```python
from build123d import *

# Parameters (mm, degrees)
BOSS_EXTRUDE1_DEPTH = 160
FILLET1_R           = 10


with BuildPart() as part:
    # Sketch1 → Boss-Extrude1 (new body)
    with BuildSketch(Plane.XY):
        with BuildLine():
            Line((0, 0), (0, -254))
            ThreePointArc((0, -254), (-1.757359313, -258.242640687), (-6, -260))
            Line((-6, -260), (-80, -260))
            Line((-80, -260), (-80, -254))
            Line((-80, -254), (-8, -254))
            ThreePointArc((-8, -254), (-6.585786438, -253.414213562), (-6, -252))
            Line((-6, -252), (-6, 0))
            Line((-6, 0), (0, 0))
        make_face()
    extrude(amount=BOSS_EXTRUDE1_DEPTH)

    # Fillet1
    fillet1_edges = [part.edges().sort_by_distance(p)[0] for p in [
        (-3, 0, 0),
        (-80, -257, 160),
        (-3, 0, 160),
        (-80, -257, 0),
    ]]
    fillet(fillet1_edges, radius=FILLET1_R)


solid = part.part
```
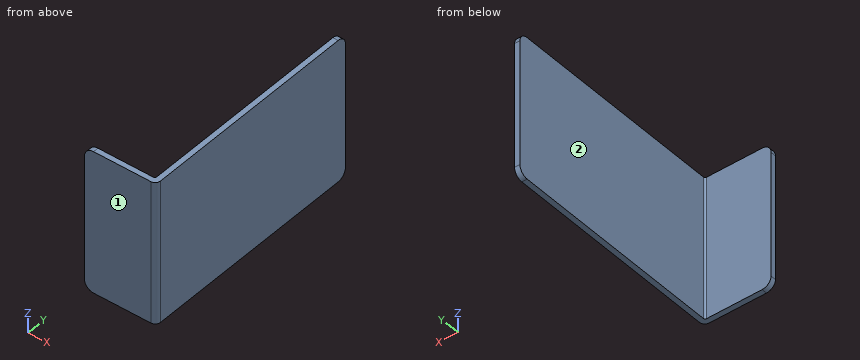
Could you check a few things on this model? Use its own coordinates, in mm. Face numbers are marked on the shaded views. A direction names the side the tool comes from. Coordinates: 2 decimals unless noted, no trailing zeros. Order: outer loops, then holes, each group sorted by start corner. A loop starts at its lowest first (then second) coordinate and runs counter-clockwise, first axis right, second up. Notation, with made-up numbers: M -16.5,-10 L -9.5,-10 A21 ccw -9.5,27 Z; hole C 1,-27.75 d4. An arc over 180 degrees is marked long. Use a Markdown table: item, result. Add a question column.
Q1. I want a section at C-C on y = -192. List the corners of the cut face in (x, z) for me.
Q2. I want a section at A-A on z = 131. List the corners of the cut face in (x, y) for me.
Q3. I'm going to push flat-ended pins straight in: pin 1 (6 mm diameter, centred on x = -70.5, z = 141, fed in from +Y); pin 2 (1.5 mm diameter, centred on y = -195, z = 100, fed in from -X). Where does each tip first touch, or does it pass through?
Q4. I want a section at B-B on x = -45.5. List the corners of the cut face in (y, z) for me, then the cut area to 3 significant figures.
Q5. Which directions (+Z, -Z, +X, -X, +Y, -Y) give clear straight access to the entire face, cutting with the end or side of a thin tool? Please do the marked faces 1 and 2.
Q6. If I drill on L1, parallel to Y at x = -35, z = 7; L2, parallel to X at y = -58.5, z = 15; L3, parallel to Y at x = -3, z = 23.5, over which ranges is the centre line in solid material (lowest first)?
Checked values:
| question | item | result |
|---|---|---|
| 1 | outline | M -6,0 L 0,0 L 0,160 L -6,160 Z |
| 2 | outline | M -80,-260 L -6,-260 A6 ccw 0,-254 L 0,0 L -6,0 L -6,-252 A2 cw -8,-254 L -80,-254 Z |
| 3 | pin 1 | y = -254 |
| 3 | pin 2 | x = -6 |
| 4 | outline | M -260,0 L -254,0 L -254,160 L -260,160 Z |
| 4 | area | 960 mm² |
| 5 | face 1 | +Z, -Z, +X, -X, -Y |
| 5 | face 2 | +Z, -Z, -X, +Y |
| 6 | L1 | -260 to -254 |
| 6 | L2 | -6 to 0 |
| 6 | L3 | -259.2 to 0 |
